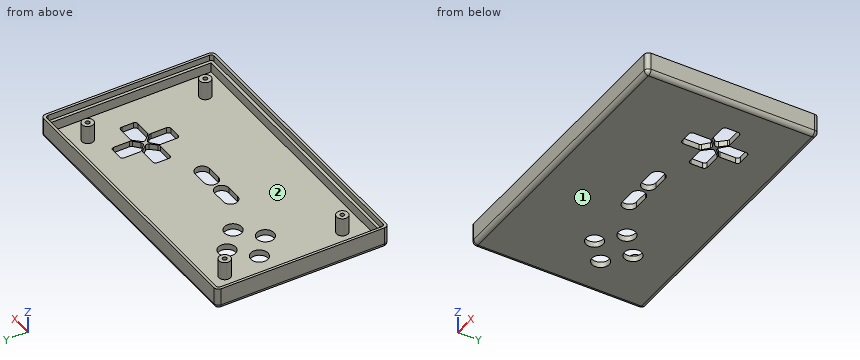
```python
from build123d import *

# Parameters (mm, degrees)
SKETCH_1_W          = 100
SKETCH_1_H          = 60
EXTRUDE_1_DEPTH     = 2
SKETCH_2_W          = 96
SKETCH_2_H          = 56
EXTRUDE_2_DEPTH     = 5.5
SKETCH_3_W          = 98.2
SKETCH_3_H          = 58.2
SKETCH_3_W_2        = 96
SKETCH_3_H_2        = 56
CUT_EXTRUDE_1_DEPTH = 2.1
FILLET_1_R          = 1.5
FILLET_2_R          = 1
SKETCH_4_R          = 2
EXTRUDE_3_DEPTH     = 6.4
SKETCH_5_R          = 0.75
CUT_EXTRUDE_3_DEPTH = 5.5
SKETCH_6_R          = 3
CUT_EXTRUDE_4_DEPTH = 10


with BuildPart() as part:
    # 草图1 → 凸台-拉伸1 (new body)
    with BuildSketch(Plane.XY):
        Rectangle(SKETCH_1_W, SKETCH_1_H)
    extrude(amount=EXTRUDE_1_DEPTH)

    # 草图2 → 凸台-拉伸2 (add)
    with BuildSketch(Plane.XY.offset(2)):
        Polygon((-48, 30), (-50, 30), (-50, 28), (-50, -28), (-50, -30), (-48, -30), (48, -30), (50, -30), (50, -28), (50, 28), (50, 30), (48, 30), align=None)
        Rectangle(SKETCH_2_W, SKETCH_2_H, mode=Mode.SUBTRACT)
    extrude(amount=EXTRUDE_2_DEPTH)

    # 草图3 → 切除-拉伸1 (cut)
    with BuildSketch(Plane.XY.offset(7.5)):
        Rectangle(SKETCH_3_W, SKETCH_3_H)
        Rectangle(SKETCH_3_W_2, SKETCH_3_H_2, mode=Mode.SUBTRACT)
    extrude(amount=-CUT_EXTRUDE_1_DEPTH, mode=Mode.SUBTRACT)

    # 圆角1
    fillet_1_edges = [part.edges().sort_by_distance(p)[0] for p in [
        (0, 30, 0),
        (50, 0, 0),
        (0, -30, 0),
        (-50, 0, 0),
        (-50, 30, 3.75),
        (50, 30, 3.75),
        (50, -30, 3.75),
        (-50, -30, 3.75),
    ]]
    fillet(fillet_1_edges, radius=FILLET_1_R)

    # 圆角2
    fillet_2_edges = [part.edges().sort_by_distance(p)[0] for p in [
        (-49.1, -29.1, 6.45),
        (-49.1, 29.1, 6.45),
        (49.1, 29.1, 6.45),
        (49.1, -29.1, 6.45),
    ]]
    fillet(fillet_2_edges, radius=FILLET_2_R)

    # 草图4 → 凸台-拉伸3 (add)
    with BuildSketch(Plane.XY.offset(2)):
        with Locations((-39, 20.5)):
            Circle(SKETCH_4_R)
        with Locations((39, 20.5)):
            Circle(SKETCH_4_R)
        with Locations((39, -20.5)):
            Circle(SKETCH_4_R)
        with Locations((-39, -20.5)):
            Circle(SKETCH_4_R)
    extrude(amount=EXTRUDE_3_DEPTH)

    # 草图5 → 切除-拉伸3 (cut)
    with BuildSketch(Plane.XY.offset(8.4)):
        with Locations((-39, 20.5)):
            Circle(SKETCH_5_R)
        with Locations((39, 20.5)):
            Circle(SKETCH_5_R)
        with Locations((39, -20.5)):
            Circle(SKETCH_5_R)
        with Locations((-39, -20.5)):
            Circle(SKETCH_5_R)
    extrude(amount=-CUT_EXTRUDE_3_DEPTH, mode=Mode.SUBTRACT)

    # 草图6 → 切除-拉伸4 (cut)
    with BuildSketch(Plane(origin=(0, 0, 0), x_dir=(-1, 0, 0), z_dir=(0, 0, -1))):
        with BuildLine():
            ThreePointArc((3, -3), (0.5, -0.5), (3, 2))
            Line((3, 2), (8, 2))
            ThreePointArc((8, 2), (10.5, -0.5), (8, -3))
            Line((8, -3), (3, -3))
        make_face()
        with Locations((21.2, 6.7)):
            Circle(SKETCH_6_R)
        with Locations((28.7, 13.4)):
            Circle(SKETCH_6_R)
        with Locations((36.2, 6.7)):
            Circle(SKETCH_6_R)
        with Locations((28.7, 0)):
            Circle(SKETCH_6_R)
        with BuildLine():
            Line((-26.039757501, 9.676852248), (-28.035430168, 7.818756103))
            ThreePointArc((-28.035430168, 7.818756103), (-28.704377925, 7.550717722), (-29.379807919, 7.801974559))
            Line((-29.379807919, 7.801974559), (-31.384135252, 9.576820114))
            ThreePointArc((-31.384135252, 9.576820114), (-31.633039063, 9.914966319), (-31.721187045, 10.325485376))
            Line((-31.721187045, 10.325485376), (-31.721187045, 15.875281781))
            ThreePointArc((-31.721187045, 15.875281781), (-31.428293826, 16.582388562), (-30.721187045, 16.875281781))
            Line((-30.721187045, 16.875281781), (-26.721187045, 16.875281781))
            ThreePointArc((-26.721187045, 16.875281781), (-26.014080264, 16.582388562), (-25.721187045, 15.875281781))
            Line((-25.721187045, 15.875281781), (-25.721187045, 10.408735966))
            ThreePointArc((-25.721187045, 10.408735966), (-25.804282049, 10.009630431), (-26.039757501, 9.676852248))
        make_face()
        with BuildLine():
            Line((-25.723147752, 4.039757501), (-27.581243897, 6.035430168))
            ThreePointArc((-27.581243897, 6.035430168), (-27.849282278, 6.704377925), (-27.598025441, 7.379807919))
            Line((-27.598025441, 7.379807919), (-25.823179886, 9.384135252))
            ThreePointArc((-25.823179886, 9.384135252), (-25.485033681, 9.633039063), (-25.074514624, 9.721187045))
            Line((-25.074514624, 9.721187045), (-19.524718219, 9.721187045))
            ThreePointArc((-19.524718219, 9.721187045), (-18.817611438, 9.428293826), (-18.524718219, 8.721187045))
            Line((-18.524718219, 8.721187045), (-18.524718219, 4.721187045))
            ThreePointArc((-18.524718219, 4.721187045), (-18.817611438, 4.014080264), (-19.524718219, 3.721187045))
            Line((-19.524718219, 3.721187045), (-24.991264034, 3.721187045))
            ThreePointArc((-24.991264034, 3.721187045), (-25.390369569, 3.804282049), (-25.723147752, 4.039757501))
        make_face()
        with BuildLine():
            Line((-31.360242499, 3.723147752), (-29.364569832, 5.581243897))
            ThreePointArc((-29.364569832, 5.581243897), (-28.695622075, 5.849282278), (-28.020192081, 5.598025441))
            Line((-28.020192081, 5.598025441), (-26.015864748, 3.823179886))
            ThreePointArc((-26.015864748, 3.823179886), (-25.766960937, 3.485033681), (-25.678812955, 3.074514624))
            Line((-25.678812955, 3.074514624), (-25.678812955, -2.475281781))
            ThreePointArc((-25.678812955, -2.475281781), (-25.971706174, -3.182388562), (-26.678812955, -3.475281781))
            Line((-26.678812955, -3.475281781), (-30.678812955, -3.475281781))
            ThreePointArc((-30.678812955, -3.475281781), (-31.385919736, -3.182388562), (-31.678812955, -2.475281781))
            Line((-31.678812955, -2.475281781), (-31.678812955, 2.991264034))
            ThreePointArc((-31.678812955, 2.991264034), (-31.595717951, 3.390369569), (-31.360242499, 3.723147752))
        make_face()
        with BuildLine():
            Line((-29.801974559, 6.020192081), (-31.576820114, 4.015864748))
            ThreePointArc((-31.576820114, 4.015864748), (-31.914966319, 3.766960937), (-32.325485376, 3.678812955))
            Line((-32.325485376, 3.678812955), (-37.875281781, 3.678812955))
            ThreePointArc((-37.875281781, 3.678812955), (-38.582388562, 3.971706174), (-38.875281781, 4.678812955))
            Line((-38.875281781, 4.678812955), (-38.875281781, 8.678812955))
            ThreePointArc((-38.875281781, 8.678812955), (-38.582388562, 9.385919736), (-37.875281781, 9.678812955))
            Line((-37.875281781, 9.678812955), (-32.408735966, 9.678812955))
            ThreePointArc((-32.408735966, 9.678812955), (-32.009630431, 9.595717951), (-31.676852248, 9.360242499))
            Line((-31.676852248, 9.360242499), (-29.818756103, 7.364569832))
            ThreePointArc((-29.818756103, 7.364569832), (-29.550717722, 6.695622075), (-29.801974559, 6.020192081))
        make_face()
        with BuildLine():
            Line((-8, 2), (-3, 2))
            ThreePointArc((-3, 2), (-0.5, -0.5), (-3, -3))
            Line((-3, -3), (-8, -3))
            ThreePointArc((-8, -3), (-10.5, -0.5), (-8, 2))
        make_face()
    extrude(amount=-CUT_EXTRUDE_4_DEPTH, mode=Mode.SUBTRACT)


solid = part.part
```
Model file for the job. Use its own axes, mm. Face numbers are marked on the shaded views. Give positions to 0.01 mm unless a question says otherwise; leave off trailing zeros. Loops run counter-clockwise (first coordinate to the right, second up) from the corner with the lowest first, then second, coordinate; pieces in that order, holes last. Notation, with made-up numbers: (-19, 55.25) - (-9, 55.25) arc R23 ccw to (-9, 75.25) - close; hole circle Ø4 at (55.5, 86.25). An arc over 180 degrees is marked (long way). One line per item, written item: value. Start each with the question number.
1. Pull direction X, two halves, no side cores. Call the marked faces 1 and 2: pulls with the +X half, pulls with the -X half, needs draft (parallel to the pull), parting line crosses it, or undercut.
2. Pin check, flat tips, straight feed: pin 1 (0.9 mm diameter, centred on x = -39, y = -20.5, fed in from +Z); pin 2 (2 mm diameter, centred on y = 6.5, z = 0.5, fed in from -X); pin 3 (1.6 mm diameter, centred on x = 35, z = 0.5, fed in from -Y); pin 4 (1.6 mm diameter, centred on x = -5, z = 0.5, fed in from +Y). Stop position of each tip, or through.
3. Slice it at B-B (z = 6.5). Give the number of separate pieces and of enclosed holes in the cut face, plus the area to 3 significant figures.
4. Slice it at A-A (x = -21.2). List the corners of the cut face in (y, z).
5. Slice it at D-D (x = 17.5). List the corners of the cut face in (y, z).
6. Probe L1, parallel to X at y = 15, z = 5; L2, parallel to X at y = 4.5, z = 1.75; L3, parallel to Y at x = 39, z = 2.5. List the from-to ranges inside material, lowest first. Write a range as from..to.
Solution:
1. face 1: needs draft
1. face 2: undercut
2. pin 1: stops at z = 2.9
2. pin 2: stops at x = -50
2. pin 3: stops at y = -29.99
2. pin 4: stops at y = 29.99
3. separate pieces: 5
3. enclosed holes: 5
3. area: 327 mm^2
4. outline: (-30, 1.5) arc R1.5 ccw to (-28.5, 0) - (3.7, 0) - (3.7, 2) - (-28, 2) - (-28, 5.4) - (-29.1, 5.4) - (-29.1, 7.5) - (-30, 7.5) - close; (9.7, 0) - (28.5, 0) arc R1.5 ccw to (30, 1.5) - (30, 7.5) - (29.1, 7.5) - (29.1, 5.4) - (28, 5.4) - (28, 2) - (9.7, 2) - close
5. outline: (-30, 1.5) arc R1.5 ccw to (-28.5, 0) - (28.5, 0) arc R1.5 ccw to (30, 1.5) - (30, 7.5) - (29.1, 7.5) - (29.1, 5.4) - (28, 5.4) - (28, 2) - (-28, 2) - (-28, 5.4) - (-29.1, 5.4) - (-29.1, 7.5) - (-30, 7.5) - close
6. L1: x = -50..-48, 48..50
6. L2: x = -50..-38.24, -34.16..-23.24, -19.16..18.55, 26.15..26.78, 30.53..31.15, 38.86..50
6. L3: y = -30..-28, -22.5..-18.5, 18.5..22.5, 28..30
